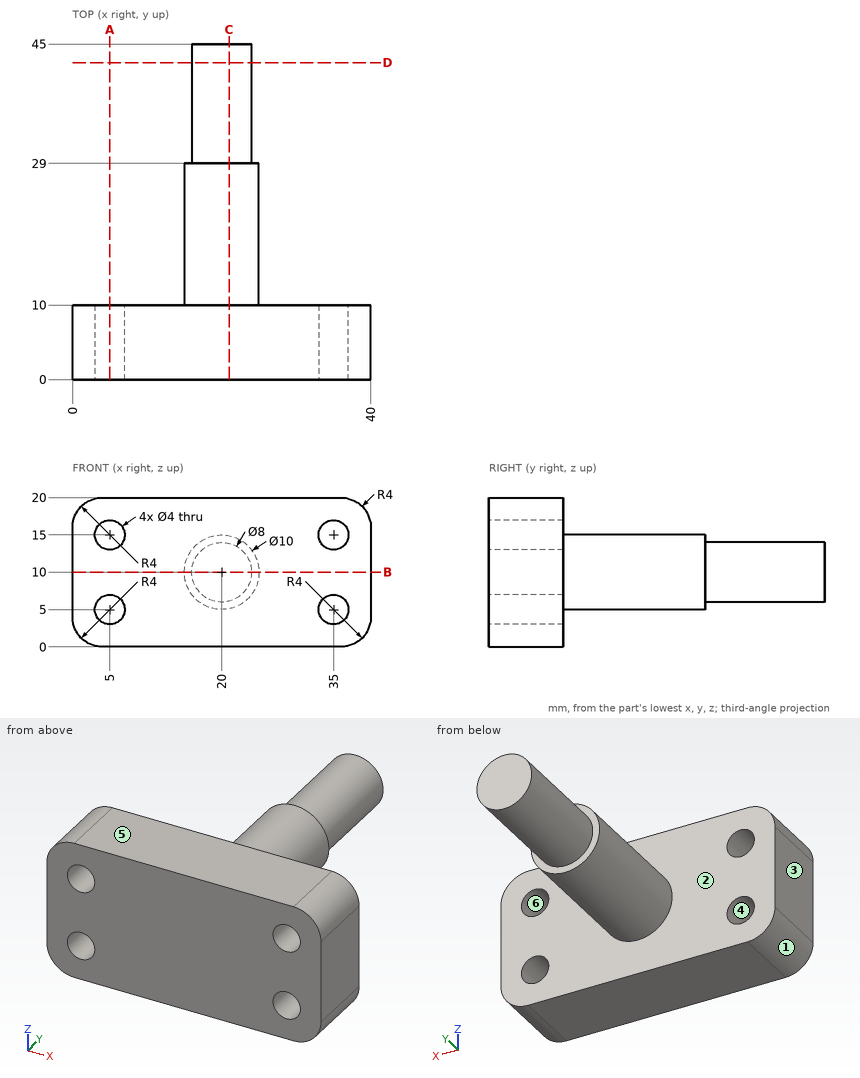
Could you check a few things on this drawing? It's one solid part, dimensions in mm from its lowest x, y, z. A direction names the side the tool comes from. Coordinates: 2 decimals unless noted, no trailing zeros. Loops run counter-clockwise (first coordinate to the right, second up) from the corner with the lowest first, then second, coordinate; pieces in that order, holes last.
1. Imagine slicing it at B-B (z = 10). Please give me the cut outline in (x, y), and give its area (3 significant figures).
2. For P1, Ø10, axis at x = 21.5, y = 21, coming from the +Z side; P2, Ø5, axis at x = 5, z = 15, coming from the +Y side; P3, Ø5, axis at y = 33, z = 12.5, coming from the +X side, each with a flat end and sliding along its axis, tell me the tip position at first contact or that it passes through.
3. Imagine slicing it at C-C (x = 21). Please give me the cut outline in (y, z).
4. We'd pull the mould along X, two halves only. Please class the marked faces 3, 4, 5 and 6: released by +X, released by -X, zero draft, split by the parting line, or undercut.
5. Imagine slicing it at A-A (x = 5). Please give me the cut outline in (y, z).
6. Imagine slicing it at D-D (y = 42.5). Please give me the cut outline in (x, z), and give its area (3 significant figures).
7. I need wall thicknesses on L1, parallel to X at y = 2, z = 5; L2, parallel to Z at x = 35, y = 6; L3, parallel to X at y = 4, z = 6.75. Which ranges of each line are inside material? Lowest first, please.
8. For the marked faces 1 and 2, which set-ups out of +Z, -Z, +X, -X, +Y, -Y let a thin tool reach every point of the face, with its end or its side?
Computed values:
1. outline: (0, 0) - (40, 0) - (40, 10) - (25, 10) - (25, 29) - (24, 29) - (24, 45) - (16, 45) - (16, 29) - (15, 29) - (15, 10) - (0, 10) - close
1. area: 718 mm2
2. P1: stops at z = 15
2. P2: stops at y = 10
2. P3: stops at x = 24
3. outline: (0, 0) - (10, 0) - (10, 5.1) - (29, 5.1) - (29, 6.13) - (45, 6.13) - (45, 13.87) - (29, 13.87) - (29, 14.9) - (10, 14.9) - (10, 20) - (0, 20) - close
4. face 3: released by -X
4. face 4: undercut
4. face 5: zero draft
4. face 6: undercut
5. outline: (0, 0) - (10, 0) - (10, 3) - (0, 3) - close; (0, 7) - (10, 7) - (10, 13) - (0, 13) - close; (0, 17) - (10, 17) - (10, 20) - (0, 20) - close
6. outline: circle Ø8 at (20, 10)
6. area: 50.3 mm2
7. L1: x = 0 to 3, 7 to 33, 37 to 40
7. L2: z = 0 to 3, 7 to 13, 17 to 20
7. L3: x = 0 to 4.03, 5.97 to 34.03, 35.97 to 40
8. face 1: -Z, -X, +Y, -Y
8. face 2: +Y
